from build123d import *

# Parameters (mm, degrees)
SKETCH1_R           = 24.5
SKETCH1_R_2         = 8
BOSS_EXTRUDE1_DEPTH = 5
SKETCH2_W           = 180
SKETCH2_H           = 100
SKETCH2_W_2         = 174
SKETCH2_H_2         = 94
BOSS_EXTRUDE2_DEPTH = 10


with BuildPart() as part:
    # Sketch1 → Boss-Extrude1 (new body)
    with BuildSketch(Plane(origin=(0, 0, 0), x_dir=(1, 0, 0), z_dir=(0, 1, 0))):
        with BuildLine():
            Line((-90, 60), (90, 60))
            ThreePointArc((90, 60), (97.071067812, 57.071067812), (100, 50))
            Line((100, 50), (100, -50))
            ThreePointArc((100, -50), (97.071067812, -57.071067812), (90, -60))
            Line((90, -60), (-90, -60))
            ThreePointArc((-90, -60), (-97.071067812, -57.071067812), (-100, -50))
            Line((-100, -50), (-100, 50))
            ThreePointArc((-100, 50), (-97.071067812, 57.071067812), (-90, 60))
        make_face()
        Circle(SKETCH1_R, mode=Mode.SUBTRACT)
        with Locations((-70, 12.5)):
            Circle(SKETCH1_R_2, mode=Mode.SUBTRACT)
        with Locations((-70, -12.5)):
            Circle(SKETCH1_R_2, mode=Mode.SUBTRACT)
        with Locations((70, 12.5)):
            Circle(SKETCH1_R_2, mode=Mode.SUBTRACT)
        with Locations((70, -12.5)):
            Circle(SKETCH1_R_2, mode=Mode.SUBTRACT)
    extrude(amount=BOSS_EXTRUDE1_DEPTH)

    # Sketch2 → Boss-Extrude2 (add)
    with BuildSketch(Plane.XZ):
        Rectangle(SKETCH2_W, SKETCH2_H)
        Rectangle(SKETCH2_W_2, SKETCH2_H_2, mode=Mode.SUBTRACT)
    extrude(amount=BOSS_EXTRUDE2_DEPTH)


solid = part.part
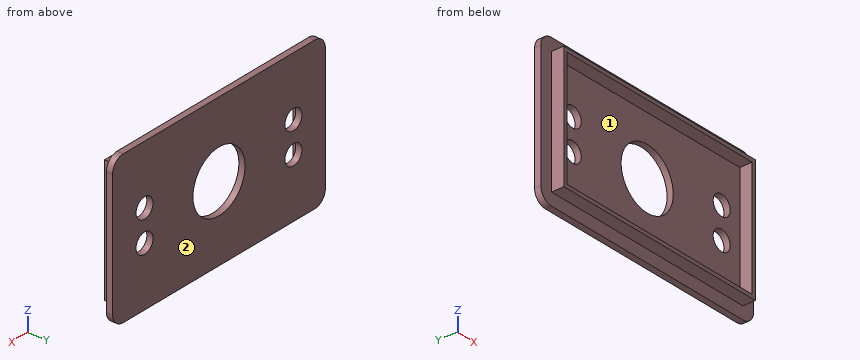
Part model, mm, in its own coordinate system. Face numbers are marked on the shaded views. Give positions to 0.01 mm unless a question says otherwise; leave off trailing zeros. Loops run counter-clockwise (first coordinate to the right, second up) from the corner with the lowest first, then second, coordinate; pieces in that order, holes last. Notation, with made-up numbers: M 85,39 L 127,39 A11 cw 127,59 Z; hole C 23.5,-7.5 d7. An arc over 180 degrees is marked long. Put each result on its own line as item: value. Start each with the question number.
1) Probe probe 1 along X at (y, z) = (2.4, 0); probe 2 along Z at (x, y) = (-70, 2.7); probe 3 along Z at (x, y) = (2, -2). List the from-to ranges inside material, lowest first.
2) Saw through at A-A (x = 0). List the corners of the cut face in (y, z), then the cut area to 3 significant figures.
3) Pull direction Z, two halves, no side cores. Call the marked faces 1 and 2: +Z half, -Z half, draft (parallel to the pull), parting line (faces both ways), or undercut.
4) Saw through at B-B (y = 2.5). List the corners of the cut face in (x, z), then the cut area to 3 significant figures.
5) Flat gauge pins, fed straight in: pin 1 (3 mm diameter, centred on x = 11.5, y = -7, fed in from -Z); pin 2 (5 mm diameter, centred on x = 25.5, y = -3.5, fed in from +Z); pin 3 (18.5 mm diameter, centred on x = -70, z = 12.5, fed in from -Y); pin 4 (13 mm diameter, centred on x = 70, z = -12.5, fed in from -Y). Where does each tip first touch, or does it go through?
6) Saw through at C-C (x = -70). List the corners of the cut face in (y, z).
7) Saw through at D-D (z = 0). List the corners of the cut face in (x, y).
Numbers:
1. probe 1: -100 to -24.5, 24.5 to 100
1. probe 2: -60 to -20.5, -4.5 to 4.5, 20.5 to 60
1. probe 3: -50 to -47, 47 to 50
2. outline: M -10,-50 L 0,-50 L 0,-60 L 5,-60 L 5,-24.5 L 0,-24.5 L 0,-47 L -10,-47 Z; M -10,47 L 0,47 L 0,24.5 L 5,24.5 L 5,60 L 0,60 L 0,50 L -10,50 Z
2. area: 415 mm^2
3. face 1: undercut
3. face 2: draft
4. outline: M -100,-50 A10 ccw -90,-60 L 90,-60 A10 ccw 100,-50 L 100,50 A10 ccw 90,60 L -90,60 A10 ccw -100,50 Z; hole C -70,-12.5 d16; hole C -70,12.5 d16; hole C 0,0 d49; hole C 70,-12.5 d16; hole C 70,12.5 d16
4. area: 21,200 mm^2
5. pin 1: z = -50
5. pin 2: z = 50
5. pin 3: y = 0
5. pin 4: through
6. outline: M -10,-50 L 0,-50 L 0,-60 L 5,-60 L 5,-20.5 L 0,-20.5 L 0,-47 L -10,-47 Z; M -10,47 L 0,47 L 0,20.5 L 5,20.5 L 5,60 L 0,60 L 0,50 L -10,50 Z; M 0,-4.5 L 5,-4.5 L 5,4.5 L 0,4.5 Z
7. outline: M -100,0 L -90,0 L -90,-10 L -87,-10 L -87,0 L -24.5,0 L -24.5,5 L -100,5 Z; M 24.5,0 L 87,0 L 87,-10 L 90,-10 L 90,0 L 100,0 L 100,5 L 24.5,5 Z
